Source: CAD feature listing. Evaluate the final solid. Frame: model axes, mm. A direction names the side the tool comes from. Round coordinates to 2 decimals unless told otherwise and drop trailing zeros. Loops run counter-clockwise (first coordinate to the right, second up) from the corner with the lowest first, then second, coordinate; pieces in that order, holes last. Notation, with made-up numbers: (-36.5, 72) -> (-20.5, 72) arc R16 ccw to (-20.5, 101) -> close; hole circle Ø4 at (65.5, 64). An arc over 180 degrees is marked (long way). Put each result on its own line as item: value. Start each with the question number.
1. Cut plane A-A (z = 5.25). Return the cut outline in (x, y), then the cut area to 3 significant figures.
2. Set-up query: faces 1 (the flat face through (0, 0, 0)), 2 (the cylindrical face through (-6.67, -5.12, 7.94)). Return all of +Z, -Z, +X, -X, +Y, -Y with unobstructed straight access to the full face (end or side cutting, diameter ignored); none if empty.
3. Material intervals for L1, parallel to Z at x = -8.75, y = 5; L2, parallel to Z at x = 1.5, y = 7.25; L3, parallel to Y at x = 0.25, z = 5.75, sorted ascending.
4. Contact query for flat-ended pins moving along their axis: pin 1 (2 mm diameter, centred on y = 0.5, z = 6.5, fed in from -X); pin 2 (8 mm diameter, centred on x = -6.5, y = 4.5, fed in from +Z) (3 decimals); pin 3 (5 mm diameter, centred on x = -4, z = 9, fed in from +Y). Output: stop coordinate, or through.
```python
from build123d import *

# Parameters (mm, degrees)
F0_W     = 23
F0_H     = 23
F1_DEPTH = 4
F2_R     = 8.408234
F3_DEPTH = 16
F4_R     = 8


with BuildPart() as f1:
    # F0 (on Top) → F1 (new body)
    with BuildSketch(Plane.XY):
        Rectangle(F0_W, F0_H)
    extrude(amount=F1_DEPTH)

    # F2 (on face) → F3 (join)
    with BuildSketch(Plane.XY.offset(4)):
        Circle(F2_R)
    extrude(amount=F3_DEPTH)

    # F4
    f4_edges = [f1.edges().sort_by_distance(p)[0] for p in [
        (-8.408234, 0, 20),
    ]]
    fillet(f4_edges, radius=F4_R)


solid = f1.part
```
Solution:
1. outline: circle Ø16.82 at (0, 0)
1. area: 222 mm^2
2. face 1: -Z, +X, -X, +Y, -Y
2. face 2: +Z
3. L1: z = 0 to 4
3. L2: z = 0 to 15.88
3. L3: y = -8.4 to 8.4
4. pin 1: stops at x = -8.41
4. pin 2: stops at z = 19.195
4. pin 3: stops at y = 8.27
